Source: CAD feature listing. Evaluate the final solid. Frame: model axes, mm. Face numbers are marked on the shaded views. A direction names the side the tool comes from. Coordinates: 2 decimals unless noted, no trailing zeros. Loops run counter-clockwise (first coordinate to the right, second up) from the corner with the lowest first, then second, coordinate; pieces in that order, holes last. Notation, with made-up numbers: (-10.5, -30.75) - (-6.5, -30.75) arc R21 ccw to (-6.5, -18.75) - close; hole circle Ø9 at (-34.5, -13). An arc over 180 degrees is marked (long way). Use one line per item in the form item = value. Start each with the question number.
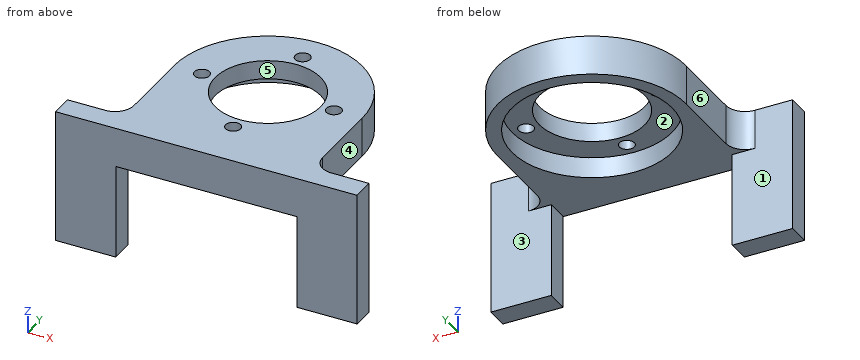
from build123d import *

# Parameters (mm, degrees)
EXTRUDE_1_DEPTH     = 10.5
SKETCH_2_R          = 14
CUT_EXTRUDE_1_DEPTH = 52.684136831
SKETCH_3_R          = 21.25
CUT_EXTRUDE_2_DEPTH = 5.5
SKETCH_4_R          = 2
CUT_EXTRUDE_3_DEPTH = 52.684136831
FILLET_1_R          = 5
SKETCH_5_W          = 16
SKETCH_5_H          = 6
EXTRUDE_2_DEPTH     = 25


with BuildPart() as part:
    # 草图1 → 凸台-拉伸1 (new body)
    with BuildSketch(Plane.XY):
        with BuildLine():
            Line((-25, 0), (-25, -25))
            Line((-25, -25), (-40, -25))
            Line((-40, -25), (-40, -31))
            Line((-40, -31), (40, -31))
            Line((40, -31), (40, -25))
            Line((40, -25), (25, -25))
            Line((25, -25), (25, 0))
            ThreePointArc((25, 0), (0, 25), (-25, 0))
        make_face()
    extrude(amount=EXTRUDE_1_DEPTH)

    # 草图2 → 切除-拉伸1 (cut, through all)
    with BuildSketch(Plane.XY.offset(10.5)):
        Circle(SKETCH_2_R)
    extrude(amount=-CUT_EXTRUDE_1_DEPTH, mode=Mode.SUBTRACT)

    # 草图3 → 切除-拉伸2 (cut)
    with BuildSketch(Plane(origin=(0, 0, 0), x_dir=(-1, 0, 0), z_dir=(0, 0, -1))):
        Circle(SKETCH_3_R)
    extrude(amount=-CUT_EXTRUDE_2_DEPTH, mode=Mode.SUBTRACT)

    # 草图4 → 切除-拉伸3 (cut, through all)
    with BuildSketch(Plane.XY.offset(10.5)):
        with Locations((0, 17.5)):
            Circle(SKETCH_4_R)
        with Locations((17.5, 0)):
            Circle(SKETCH_4_R)
        with Locations((0, -17.5)):
            Circle(SKETCH_4_R)
        with Locations((-17.5, 0)):
            Circle(SKETCH_4_R)
    extrude(amount=-CUT_EXTRUDE_3_DEPTH, mode=Mode.SUBTRACT)

    # 圆角1
    fillet_1_edges = [part.edges().sort_by_distance(p)[0] for p in [
        (25, -25, 5.25),
        (-25, -25, 5.25),
    ]]
    fillet(fillet_1_edges, radius=FILLET_1_R)

    # 草图5 → 凸台-拉伸2 (add)
    with BuildSketch(Plane(origin=(0, 0, 0), x_dir=(-1, 0, 0), z_dir=(0, 0, -1))):
        with Locations((32, -28)):
            Rectangle(SKETCH_5_W, SKETCH_5_H)
        with Locations((-32, -28)):
            Rectangle(SKETCH_5_W, SKETCH_5_H)
    extrude(amount=EXTRUDE_2_DEPTH)


solid = part.part
(1) Cut plane C-C, the plane x = -17.5. Output: boundary loops of the cut face in (y, z).
(2) Cut plane B-B, the plane z = -7.5. Output: boundary loops of the cut face in (x, y).
(3) Mould query, pull axis X, two halves, no side actions, for the marked faces 4, 5 and 6. Classes: +X half, -X half, draft (parallel to the pull), parting line (faces both ways), or undercut.
(4) Cut plane D-D, the plane y = 17.5. Output: boundary loops of the cut face in (x, z).
(5) Access query for the marked faces 1, 2 and 3. Directions: +Z, -Z, +X, -X, +Y, -Y. A direction counts if a zero-diameter tool reaches every point of the face in a straight line with its end or side. Return the directions, or none.
(6) Contact query for flat-ended pins moving along their axis: pin 1 (5 mm diameter, centred on y = -12.5, z = 7, fed in from +X); pin 2 (11.5 mm diameter, centred on y = -6, z = 5.5, fed in from -X); pin 3 (17 mm diameter, centred on x = 11, y = -8.5, fed in from -Z). Output: stop coordinate, or through.
(7) Material intervals for line 1 (Y direction, x = 0, z = 8); line 2 (Y direction, x = 0, z = 2.95); line 3 (X direction, y = 9, z = 2), sorted ascending.
(8) Cut plane A-A, the plane x = 0. Output: boundary loops of the cut face in (y, z), plus the area to 3 significant figures.
Recorded:
q1.outline = (-31, 0) - (-12.05, 0) - (-12.05, 5.5) - (-2, 5.5) - (-2, 10.5) - (-31, 10.5) - close; (2, 5.5) - (12.05, 5.5) - (12.05, 0) - (17.85, 0) - (17.85, 10.5) - (2, 10.5) - close
q2.outline = (-40, -31) - (-24, -31) - (-24, -25) - (-40, -25) - close; (24, -31) - (40, -31) - (40, -25) - (24, -25) - close
q3.face_4 = +X half
q3.face_5 = undercut
q3.face_6 = -X half
q4.outline = (-17.85, 0) - (-12.05, 0) - (-12.05, 5.5) - (-2, 5.5) - (-2, 10.5) - (-17.85, 10.5) - close; (2, 5.5) - (12.05, 5.5) - (12.05, 0) - (17.85, 0) - (17.85, 10.5) - (2, 10.5) - close
q5.face_1 = -Z, -X, +Y
q5.face_2 = -Z
q5.face_3 = -Z, +X, +Y
q6.pin_1 = 25
q6.pin_2 = -25
q6.pin_3 = 0
q7.line_1 = -31 to -19.5, -15.5 to -14, 14 to 15.5, 19.5 to 25
q7.line_2 = -31 to -21.25, 21.25 to 25
q7.line_3 = -23.32 to -19.25, 19.25 to 23.32
q8.outline = (-31, 0) - (-21.25, 0) - (-21.25, 5.5) - (-19.5, 5.5) - (-19.5, 10.5) - (-31, 10.5) - close; (-15.5, 5.5) - (-14, 5.5) - (-14, 10.5) - (-15.5, 10.5) - close; (14, 5.5) - (15.5, 5.5) - (15.5, 10.5) - (14, 10.5) - close; (19.5, 5.5) - (21.25, 5.5) - (21.25, 0) - (25, 0) - (25, 10.5) - (19.5, 10.5) - close
q8.area = 174 mm²
